```python
from build123d import *

# Parameters (mm, degrees)
SKETCH2_W          = 7
SKETCH2_H          = 1
SKETCH3_R          = 3.05
CUT_EXTRUDE1_DEPTH = 57.789083458
CHAMFER1_SIZE      = 2
SKETCH4_R          = 9
CUT_EXTRUDE2_DEPTH = 57.648036153
SKETCH5_R          = 1.6
CUT_EXTRUDE3_DEPTH = 57.789083458


with BuildPart() as part:
    # Sketch2 → Revolve1 (revolve)
    with BuildSketch(Plane(origin=(0, 0, 0), x_dir=(1, 0, 0), z_dir=(0, 1, 0))):
        with Locations((3.5, -2.5)):
            Rectangle(SKETCH2_W, SKETCH2_H)
        with BuildLine():
            Line((0, 2), (0, -2))
            Line((0, -2), (7, -2))
            Line((7, -2), (7, -1))
            Line((7, -1), (35.767949192, -1))
            Line((35.767949192, -1), (37.5, -2))
            Line((37.5, -2), (40, -2))
            Line((40, -2), (40, -1))
            ThreePointArc((40, -1), (39, 0), (40, 1))
            Line((40, 1), (40, 2))
            Line((40, 2), (0, 2))
        make_face()
    revolve(axis=Axis((0, 0, 2), (0, 0, -1)))

    # Sketch3 → Cut-Extrude1 (cut, through all)
    with BuildSketch(Plane.XY.offset(3)):
        Circle(SKETCH3_R)
    extrude(amount=-CUT_EXTRUDE1_DEPTH, mode=Mode.SUBTRACT)

    # Chamfer1
    chamfer1_edges = [part.edges().sort_by_distance(p)[0] for p in [
        (-7, 0, 1),
    ]]
    chamfer(chamfer1_edges, length=CHAMFER1_SIZE - 0.0001)  # a hair under: the kernel refuses the full size

    # Sketch4 → Cut-Extrude2 (cut, through all)
    with BuildSketch(Plane.XY.offset(1)):
        with Locations((0, -22)):
            Circle(SKETCH4_R)
        with Locations((-20.923243358, -6.798373876)):
            Circle(SKETCH4_R)
        with Locations((-12.93127555, 17.798373876)):
            Circle(SKETCH4_R)
        with Locations((12.93127555, 17.798373876)):
            Circle(SKETCH4_R)
        with Locations((20.923243358, -6.798373876)):
            Circle(SKETCH4_R)
    extrude(amount=-CUT_EXTRUDE2_DEPTH, mode=Mode.SUBTRACT)

    # Sketch5 → Cut-Extrude3 (cut, through all)
    with BuildSketch(Plane(origin=(0, 0, -2), x_dir=(-1, 0, 0), z_dir=(0, 0, -1))):
        with Locations((0, 12)):
            Circle(SKETCH5_R)
        with Locations((0, 32)):
            Circle(SKETCH5_R)
    extrude(amount=-CUT_EXTRUDE3_DEPTH, mode=Mode.SUBTRACT)


solid = part.part
```
Input: part model. Units: mm. Frame: model coordinates. A direction names the side the tool comes from. Round coordinates to 2 decimals unless told otherwise and drop trailing zeros. Write each question's results on one line, items separated by ' | '.
Q1. Access query for faces 1 (the face through (0.208, 13.586, -0.521)), 2 (the face through (-7, -8, 1)). Directions: +Z, -Z, +X, -X, +Y, -Y. A direction counts if a zero-diameter tool reaches every point of the face in a straight line with its end or side. Return the directions, or none.
Results:
face 1: +Z, -Z | face 2: +Z
Q2. Draft query along X for faces 3 (the face through (-8.67, 39.05, -1.51)), 4 (the face through (-1.54, 6.96, 2.87)), 5 (the face through (-1.5, 3, 3)). Return one class per face: released by +X, released by -X, zero draft, split by the parting line, or undercut.
Results:
face 3: split by the parting line | face 4: undercut | face 5: zero draft
Q3. Line query: line 1 along Y through (x, z) = (0, -1.1); line 2 along Y through (x, z) = (21, -1.6); line 3 along Y through (x, z) = (0, 0.15). Output: solid intervals per line, ascending.
Results:
line 1: y = -40 to -31, -13 to -3.05, 3.05 to 10.4, 13.6 to 30.4, 33.6 to 40 | line 2: y = -34.04 to -15.8, 2.2 to 13.81, 21.79 to 34.04 | line 3: y = -39.01 to -31, -13 to -3.05, 3.05 to 10.4, 13.6 to 30.4, 33.6 to 39.01
Q4. Section query A-A (x = 0). State how many separate pieces and enclosed holes the cut face has, and give its area (3 significant figures).
Results:
separate pieces: 5 | enclosed holes: 0 | area: 172 mm^2
Q5. Pin query (flat end, axial travel): P1, Ø8, axis at x = -14, y = 2, coming from the +Z side; P2, Ø10, axis at x = 31.5, y = 4, coming from the +Z side; P3, Ø2, axis at x = -12, z = -1.5, coming from the -Y side. Return the tip coordinate at first contact, or that it passes through.
Results:
P1: stops at z = 1 | P2: stops at z = 1.57 | P3: stops at y = -38.46
